Input: part model. Units: mm. Frame: model coordinates. A direction names the side the tool comes from. Give positions to 0.01 mm unless a question says otherwise; leave off trailing zeros. Write each loop counter-clockwise with the first axis right and the second up, starting at its lowest first coordinate (ties: lowest second). Pieces come first, ordered by that corner, then holes. Notation, with made-up numbers: M 89.5,53 L 100.5,53 A11 ccw 100.5,66 Z; hole C -33,52.5 d2. An arc over 180 degrees is marked long. Use CSV: the item, a comma, the result in double quotes. Start each with the question number.
Autodesk Inventor part; units mm, degrees
ref_plane "YZ Plane" through (0, 0, 0) normal (1, 0, 0) x (0, 1, 0)
ref_plane "XZ Plane" through (0, 0, 0) normal (0, 1, 0) x (-1, 0, 0)
ref_plane "XY Plane" through (0, 0, 0) normal (0, 0, 1) x (1, 0, 0)
sketch "Sketch1" plane through (0, 0, 0) normal (1, 0, 0) x (0, 1, 0)
  line L0 (60.8092, 49.7341) -> (-41.1908, 49.7341)
  line L1 (-41.1908, 49.7341) -> (-41.1908, -72.2659)
  line L2 (-41.1908, -72.2659) -> (60.8092, -72.2659)
  line L3 (60.8092, -72.2659) -> (60.8092, 49.7341)
  point P0 (0, 0)
  dimension "d0" = 122
  dimension "d1" = 102
extrude "Extrusion1" add sketch "Sketch1" along normal blind 5.08
sketch "Sketch2" plane through (5.08, 0, 0) normal (1, 0, 0) x (0, 0, -1)
  line L0 (-49.7341, 60.8092) -> (-49.7341, -41.1908)
  line L1 (72.2659, 60.8092) -> (-49.7341, 60.8092)
  point P0 (0, 0)
  point P1 (-35.7341, 46.8092)
  point P2 (50.2659, 46.8092)
  point P3 (50.2659, -11.1908)
  point P4 (-35.7341, -11.1908)
  dimension "d5" = 0
  dimension "d15" = 14
  dimension "d16" = 14
  dimension "d17" = 0
  dimension "d18" = 72
  dimension "d19" = 100
  dimension "d20" = 0
  dimension "d21" = 0
hole "Hole1" at (5.08, 46.8092, 35.7341) at (5.08, 46.8092, -50.2659) at (5.08, -11.1908, -50.2659) at (5.08, -11.1908, 35.7341) direction (-1, 0, 0) diameter 2.0574 end through all
sketch "Sketch3" plane through (5.08, 0, 0) normal (1, 0, 0) x (0, 0, -1)
  circle A0 centre (-35.7341, 46.8092) radius 1.0287
  circle A1 centre (-35.7341, 46.8092) radius 2.54
  circle A2 centre (50.2659, 46.8092) radius 1.0287
  circle A3 centre (50.2659, 46.8092) radius 2.54
  circle A4 centre (50.2659, -11.1908) radius 1.0287
  circle A5 centre (50.2659, -11.1908) radius 2.54
  circle A6 centre (-35.7341, -11.1908) radius 1.0287
  circle A7 centre (-35.7341, -11.1908) radius 2.54
  point P0 (0, 0)
  dimension "d22" = 5.08
  dimension "d23" = 5.08
  dimension "d24" = 5.08
  dimension "d25" = 5.08
extrude "Extrusion2" add sketch "Sketch3" along normal blind 5.08
sketch "Sketch4" plane through (5.08, 0, 0) normal (1, 0, 0) x (0, 0, -1)
  line L0 (-49.7341, 60.8092) -> (-49.7341, -41.1908)
  line L1 (72.2659, 60.8092) -> (-49.7341, 60.8092)
  point P0 (0, 0)
  point P1 (-43.3841, 54.4592)
  point P2 (65.8359, 54.4592)
  point P3 (-43.3841, -34.4408)
  point P4 (65.8359, -34.4408)
  dimension "d28" = 6.35
  dimension "d29" = 6.35
  dimension "d30" = 109.22
  dimension "d31" = 0
  dimension "d32" = 88.9
  dimension "d33" = 0
  dimension "d34" = 0
  dimension "d35" = 0
hole "Hole2" at (5.08, 54.4592, 43.3841) at (5.08, 54.4592, -65.8359) at (5.08, -34.4408, 43.3841) at (5.08, -34.4408, -65.8359) direction (-1, 0, 0) diameter 5.1054 end through all
properties part number "JetsonPlate"
Q1. Section C-C, the plane z = -24.5. Return the cut outline in (x, y), and give its area (3 significant figures).
Q2. Material intervals for L1, parallel to X at y = 44.5, z = -56; L2, parallel to Z at x = 3.75, y = 56, sorted ascending. Write a range as [from, to].
Q3. First-contact query: pin 1 Ø1.2 at (y, z) = (46.81, 35.73) entering from +X. Flat tip, straight axial feed; report the tip coordinate or a pass-through.
Q4. Section A-A, the plane x = 7. Return the cut outline in (y, z), and give its area (3 significant figures).
Q5. Section B-B, the plane y = 21.5. Return the cut outline in (x, z), and give its area (3 significant figures).
Q6. Pull-direction query (Z, two-part tool) for faces 1 (the flat face through (3, 11, 49.734)), 2 (the flat face through (10.16, -11.7, -51.4)), 3 (the flat face through (3, 9, -72.266)), 4 (the cylindrical face through (7.58, 46.05, -52.69)); classes: released by +Z, released by -Z, zero draft, split by the parting line, or undercut.
Q7. Set-up query: faces 5 (the flat face through (3, -41.191, -10)), 6 (the cylindrical face through (7.584, -10.218, -52.612)). Return all of +Z, -Z, +X, -X, +Y, -Y with unobstructed straight access to the full face (end or side cutting, diameter ignored); none if empty.
Check result:
1,outline,"M 0,-41.19 L 5.08,-41.19 L 5.08,60.81 L 0,60.81 Z"
1,area,"518 mm²"
2,L1,"x = [0, 5.08]"
2,L2,"z = [-72.27, -67.87], [-63.8, 41.35], [45.42, 49.73]"
3,pin 1,"passes through"
4,outline,"C -11.19,-50.27 d5.08; C -11.19,35.73 d5.08; C 46.81,-50.27 d5.08; C 46.81,35.73 d5.08; hole C -11.19,-50.27 d2.06; hole C -11.19,35.73 d2.06; hole C 46.81,-50.27 d2.06; hole C 46.81,35.73 d2.06"
4,area,"67.8 mm²"
5,outline,"M 0,-72.27 L 5.08,-72.27 L 5.08,49.73 L 0,49.73 Z"
5,area,"620 mm²"
6,face 1,"released by +Z"
6,face 2,"zero draft"
6,face 3,"released by -Z"
6,face 4,"undercut"
7,face 5,"+Z, -Z, +X, -X, -Y"
7,face 6,"+X"
